Source: CAD feature listing. Evaluate the final solid. Frame: model axes, mm. Face numbers are marked on the shaded views. A direction names the side the tool comes from. Round coordinates to 2 decimals unless told otherwise and drop trailing zeros. Order: outer loops, then holes, each group sorted by start corner. A loop starts at its lowest first (then second) coordinate and runs counter-clockwise, first axis right, second up. Notation, with made-up numbers: (71.25, 67.5) -> (96.25, 67.5) arc R28 cw to (96.25, 89.5) -> close; hole circle Ø3 at (-13.75, 66). An arc over 180 degrees is marked (long way). Use a Markdown table: item, result. Add a question column.
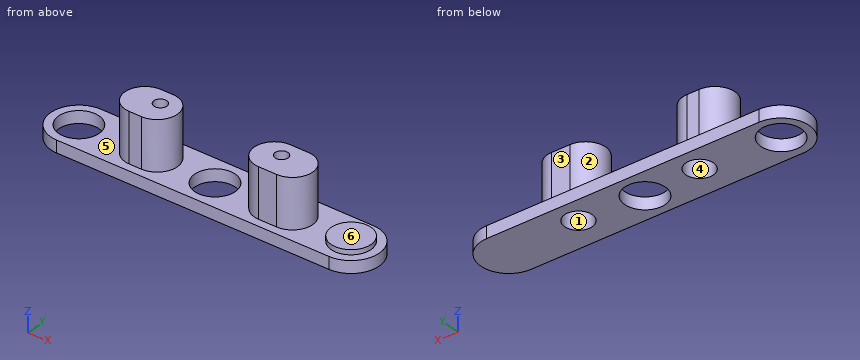
```python
from build123d import *

# Parameters (mm, degrees)
PAD008_DEPTH    = 3
PAD009_DEPTH    = 15.2
SKETCH025_R     = 5.05
SKETCH025_R_2   = 1.6
POCKET_DEPTH    = 15.2
SKETCH026_R     = 4.95
PAD010_DEPTH    = 1.2
SKETCH027_R     = 3.45
POCKET001_DEPTH = 13


with BuildPart() as leftdrivegearretainerbody:
    # Sketch023 → Pad008 (new body)
    with BuildSketch(Plane.XY.offset(12.2)):
        with BuildLine():
            ThreePointArc((-67.387162, 7), (-74.387162, 0), (-67.387162, -7))
            Line((-67.387162, -7), (0, -7))
            ThreePointArc((0, -7), (7, 0), (0, 7))
            Line((-67.387162, 7), (0, 7))
        make_face()
    extrude(amount=PAD008_DEPTH)

    # Sketch024 → Pad009 (join)
    with BuildSketch(Plane.XY):
        with BuildLine():
            ThreePointArc((-19, 5), (-24, 0), (-19, -5))
            Line((-19, -5), (-14.5, -5))
            ThreePointArc((-14.5, -5), (-9.5, 0), (-14.5, 5))
            Line((-19, 5), (-14.5, 5))
        make_face()
        with BuildLine():
            ThreePointArc((-51, 5), (-56, 0), (-51, -5))
            Line((-51, -5), (-48, -5))
            ThreePointArc((-48, -5), (-43, 0), (-48, 5))
            Line((-51, 5), (-48, 5))
        make_face()
    extrude(amount=PAD009_DEPTH)

    # Sketch025 → Pocket (cut)
    with BuildSketch(Plane.XY):
        with Locations((-33.693581, 0)):
            Circle(SKETCH025_R)
        with Locations((-67.387162, 0)):
            Circle(SKETCH025_R)
        with Locations((-18, 1)):
            Circle(SKETCH025_R_2)
        with Locations((-48, 1)):
            Circle(SKETCH025_R_2)
    extrude(amount=POCKET_DEPTH, mode=Mode.SUBTRACT)

    # Sketch026 → Pad010 (join)
    with BuildSketch(Plane.XY.offset(12.2)):
        Circle(SKETCH026_R)
    extrude(amount=-PAD010_DEPTH)

    # Sketch027 → Pocket001 (cut)
    with BuildSketch(Plane.XY.offset(15.2)):
        with Locations((-18, 1)):
            Circle(SKETCH027_R)
        with Locations((-48, 1)):
            Circle(SKETCH027_R)
    extrude(amount=-POCKET001_DEPTH, mode=Mode.SUBTRACT)


with BuildPart() as rightdrivegearretainer:
    # Part__Mirroring004: instance of LeftDriveGearRetainerBody
    add(leftdrivegearretainerbody.part.mirror(Plane(origin=(0, 0, 0), x_dir=(0, 1, 0), z_dir=(0, 0, 1))))


solid = rightdrivegearretainer.part
```
1) Section A-A on z = -9. Output: boundary loops of the cut face in (x, y).
2) Draft query along Y for the marked faces 1, 2 and 3. Return one class per face: pulls with the +Y half, pulls with the -Y half, needs draft (parallel to the pull), parting line crosses it, or undercut.
3) Reachability of the marked faces 4, 5 and 6 from +Z, -Z, +X, -X, +Y, -Y: full face, straight path, thin tool, end or side. Return the list, or none.
4) First-contact query: pin 1 Ø3 at (x, y) = (-1.5, 0.5) entering from +Z; pin 2 Ø1.5 at (x, z) = (-17, -4.5) entering from +Y; pin 3 Ø1.5 at (x, z) = (-50, -3.5) entering from -Y; pin 4 Ø8 at (x, z) = (-18, -9.5) entering from +Y. Flat tips, straight axial feed; report the tip coordinate or a pass-through.
5) Section C-C on z = -13.75. Output: boundary loops of the cut face in (x, y), then the cut area to 3 significant figures.
6) Line query: probe 1 along Y at (x, z) = (-18, -1.7); probe 2 along X at (y, z) = (0, -14.15); probe 3 along Y at (x, z) = (-48, -9.25). Output: solid intervals per line, ascending. Write a range as from..to.
7) Section D-D on y = -1.5. Count the separate pieces of the cut face and the enclosed holes in it, then the cut area to 3 significant figures.
8) Section B-B on x = -18. Output: boundary loops of the cut face in (y, z).
Conclusion:
| question | item | result |
|---|---|---|
| 1 | outline | (-51, -5) -> (-48, -5) arc R5 ccw to (-48, 5) -> (-51, 5) arc R5 ccw to start; (-19, -5) -> (-14.5, -5) arc R5 ccw to (-14.5, 5) -> (-19, 5) arc R5 ccw to start; hole circle Ø6.9 at (-48, 1); hole circle Ø6.9 at (-18, 1) |
| 2 | face 1 | undercut |
| 2 | face 2 | parting line crosses it |
| 2 | face 3 | pulls with the +Y half |
| 3 | face 4 | -Z |
| 3 | face 5 | +Z |
| 3 | face 6 | +Z, +X, +Y, -Y |
| 4 | pin 1 | stops at z = -11 |
| 4 | pin 2 | stops at y = 5 |
| 4 | pin 3 | stops at y = -5 |
| 4 | pin 4 | stops at y = 7 |
| 5 | outline | (-67.39, -7) -> (0, -7) arc R7 ccw to (0, 7) -> (-67.39, 7) arc R7 ccw to start; hole circle Ø10.1 at (-67.39, 0); hole circle Ø6.9 at (-48, 1); hole circle Ø10.1 at (-33.69, 0); hole circle Ø6.9 at (-18, 1) |
| 5 | area | 862 mm^2 |
| 6 | probe 1 | y = -5..-0.6, 2.6..5 |
| 6 | probe 2 | x = -74.39..-72.44, -62.34..-51.3, -44.7..-38.74, -28.64..-21.3, -14.7..7 |
| 6 | probe 3 | y = -5..-2.45, 4.45..5 |
| 7 | separate pieces | 3 |
| 7 | enclosed holes | 0 |
| 7 | area | 397 mm^2 |
| 8 | outline | (-7, -15.2) -> (-2.45, -15.2) -> (-2.45, -2.2) -> (-0.6, -2.2) -> (-0.6, 0) -> (-5, 0) -> (-5, -12.2) -> (-7, -12.2) -> close; (2.6, -2.2) -> (4.45, -2.2) -> (4.45, -15.2) -> (7, -15.2) -> (7, -12.2) -> (5, -12.2) -> (5, 0) -> (2.6, 0) -> close |
